from build123d import *

# Parameters (mm, degrees)
SKETCH_R   = 2.65
SKETCH_R_2 = 1.65
PAD_DEPTH  = 5


with BuildPart() as part:
    # Sketch → Pad (new body)
    with BuildSketch(Plane.XY):
        Polygon((-120, 20), (18, 20), (18, -80), (0, -80), (-120, 0), align=None)
        with Locations((-10, 10)):
            Circle(SKETCH_R, mode=Mode.SUBTRACT)
        with Locations((-110, 10)):
            Circle(SKETCH_R, mode=Mode.SUBTRACT)
        with Locations((-70, 10)):
            Circle(SKETCH_R, mode=Mode.SUBTRACT)
        with Locations((-30, 10)):
            Circle(SKETCH_R, mode=Mode.SUBTRACT)
        with Locations((10, 15)):
            Circle(SKETCH_R_2, mode=Mode.SUBTRACT)
        with Locations((10, -20)):
            Circle(SKETCH_R_2, mode=Mode.SUBTRACT)
        with Locations((10, -40)):
            Circle(SKETCH_R_2, mode=Mode.SUBTRACT)
        with Locations((10, -75)):
            Circle(SKETCH_R_2, mode=Mode.SUBTRACT)
    extrude(amount=PAD_DEPTH)


solid = part.part
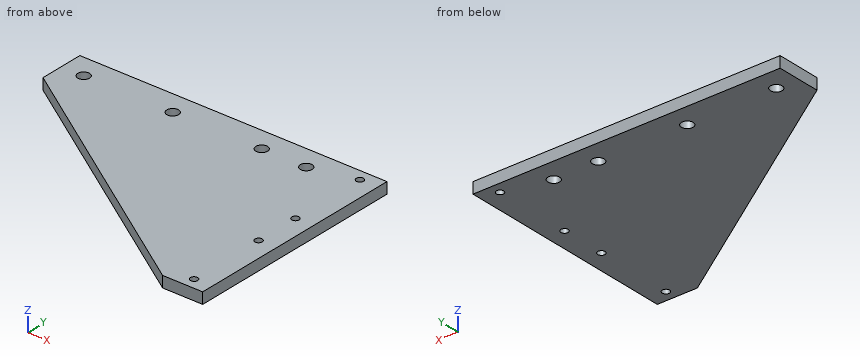
The listing builds one solid part. Answer for the finished solid, in the listing's coordinates (mm). Coordinates: 2 decimals unless noted, no trailing zeros. Order: outer loops, then holes, each group sorted by start corner. A loop starts at its lowest first (then second) coordinate and runs counter-clockwise, first axis right, second up.
Q1. Given P1, Ø8.5, axis at x = -30, y = 10, coming from the -Z side; P2, Ø1.5, axis at x = -80.5, z = 1.5, coming from the -Y side; P3, Ø3, axis at x = -10, y = 10, coming from the +Z side, each flat-ended and moving along its own axis, determine where each tip first touches the part or whether it passes through.
Q2. A cutting plane is placed at D-D, the plane x = -30. Write down the section's boundary in (y, z), and give its area (4 significant figures).
Q3. A cutting plane is placed at A-A, the plane y = 15. Write down the section's boundary in (x, z), and give its area (4 significant figures).
Q4. A cutting plane is placed at B-B, the plane x = 10. Write down the section's boundary in (y, z).
Q5. A cutting plane is placed at C-C, the plane z = 1.4. State how many separate pieces and enclosed holes the cut face has, and give its area (3 significant figures).
Q6. Consider line 1 (Y direction, x = 10, z = 1.35); line 2 (Y direction, x = -10, z = 1.6); line 3 (Y direction, x = -70, z = 3.8). Determine where each line is inside the solid, lowest interval first.
Answers follow:
1. P1: stops at z = 0
1. P2: stops at y = -26.83
1. P3: passes through
2. outline: (-60, 0) - (7.35, 0) - (7.35, 5) - (-60, 5) - close; (12.65, 0) - (20, 0) - (20, 5) - (12.65, 5) - close
2. area: 373.5 mm2
3. outline: (-120, 0) - (8.35, 0) - (8.35, 5) - (-120, 5) - close; (11.65, 0) - (18, 0) - (18, 5) - (11.65, 5) - close
3. area: 673.5 mm2
4. outline: (-80, 0) - (-76.65, 0) - (-76.65, 5) - (-80, 5) - close; (-73.35, 0) - (-41.65, 0) - (-41.65, 5) - (-73.35, 5) - close; (-38.35, 0) - (-21.65, 0) - (-21.65, 5) - (-38.35, 5) - close; (-18.35, 0) - (13.35, 0) - (13.35, 5) - (-18.35, 5) - close; (16.65, 0) - (20, 0) - (20, 5) - (16.65, 5) - close
5. separate pieces: 1
5. enclosed holes: 8
5. area: 8,880 mm2
6. line 1: y = -80 to -76.65, -73.35 to -41.65, -38.35 to -21.65, -18.35 to 13.35, 16.65 to 20
6. line 2: y = -73.33 to 7.35, 12.65 to 20
6. line 3: y = -33.33 to 7.35, 12.65 to 20
